Part model, mm, in its own coordinate system. A direction names the side the tool comes from. Coordinates: 2 decimals unless noted, no trailing zeros. Loops run counter-clockwise (first coordinate to the right, second up) from the corner with the lowest first, then second, coordinate; pieces in that order, holes last. Notation, with made-up numbers: (-38, 76.25) - (10, 76.25) arc R11 ccw to (10, 94.25) - close; hole circle Ø5 at (-16.5, 47.5). An arc over 180 degrees is marked (long way). Use a Markdown table: item, result. Add a question column.
1. 3-axis set-ups, long thin cutter, end or side, ignore diameter. For faces 5 (the flat face through (-19, -1, -12.8)), 6 (the flat face through (-20, -1, -36)), 7 (the flat face through (-1, -1, -6.4)): which of +Z, -Z, +X, -X, +Y, -Y reach the whole face in a straight line?
2. Band-saw the part on D-D, the plane z = -8. Give the cut face in (x, y), plus the area to 4 significant figures.
3. Band-saw the part on A-A, the plane z = -17.7. Give the cut face in (x, y).
4. Wall check: probe 1 along X at (y, z) = (-0.85, -30.5); probe 2 along Y at (x, z) = (-10, 0.8); probe 3 along Z at (x, y) = (-5, 7). Give the ranges that are in metal, low to high. Write a range as [from, to].
5. Band-saw the part on C-C, the plane x = -17.5. Count the separate pieces of the cut face and the enclosed holes in it, plus the area to 3 significant figures.
6. Band-saw the part on B-B, the plane y = 17. Give the cut face in (x, z), plus the area to 3 significant figures.
7. Pull direction Z, two halves, no side cores. Call faces 1 (the cylindrical face through (-3.65, -0.74, -33.56)), 2 (the flat face through (-10, 6, 1.5)), 3 (the cylindrical face through (-10, 20, 1)), 4 (the flat face through (-10, -1, -40)): pulls with the +Z half, pulls with the -Z half, needs draft (parallel to the pull), parting line crosses it, or undercut.
8. Drop flat-ended pins along their axis: pin 1 (1.6 mm diameter, centred on x = -1, y = -1, fed in from +Z); pin 2 (6 mm diameter, centred on x = -13, y = 11.5, fed in from -Z); pin 3 (0.8 mm diameter, centred on x = -0.5, y = -1, fed in from -Z). Give the stop position or say it passes through.
from build123d import *

# Parameters (mm, degrees)
BOSS_EXTRUDE1_DEPTH  = 20
CUT_EXTRUDE2_DEPTH   = 20
CUT_EXTRUDE3_DEPTH   = 20
SKETCH4_R            = 3.75
CUT_EXTRUDE4_DEPTH   = 20
SKETCH5_R            = 1.45
CUT_EXTRUDE5_DEPTH   = 20
CIRPATTERN1_COUNT    = 4
SKETCH6_R            = 1.6
CUT_EXTRUDE6_DEPTH   = 20
LPATTERN1_COUNT      = 6
LPATTERN1_PITCH      = 6.4
CUT_EXTRUDE7_DEPTH   = 20
LPATTERN2_COUNT      = 5
LPATTERN2_PITCH      = 6.4
MIRROR1_COPY_1_DEPTH = 20
MIRROR1_COPY_2_DEPTH = 20
MIRROR1_COPY_3_DEPTH = 20
MIRROR1_COPY_4_DEPTH = 20
FILLET3_R            = 3.65
FILLET4_R            = 3.65


with BuildPart() as part:
    # Sketch1 → Boss-Extrude1 (new body)
    with BuildSketch(Plane(origin=(0, 0, 0), x_dir=(0, 0, -1), z_dir=(1, 0, 0))):
        Polygon((0, 0), (0, 20), (-1.5, 20), (-1.5, -1.5), (40, -1.5), (40, 0), align=None)
    extrude(amount=-BOSS_EXTRUDE1_DEPTH)

    # Sketch2 → Cut-Extrude2 (cut)
    with BuildSketch(Plane(origin=(0, 0, 0), x_dir=(0, 0, -1), z_dir=(1, 0, 0))):
        with BuildLine():
            Line((-1.5, 0), (-1.5, -1.5))
            Line((-1.5, -1.5), (0, -1.5))
            ThreePointArc((0, -1.5), (-1.060660172, -1.060660172), (-1.5, 0))
        make_face()
    extrude(amount=-CUT_EXTRUDE2_DEPTH, mode=Mode.SUBTRACT)

    # Sketch3 → Cut-Extrude3 (cut)
    with BuildSketch(Plane.XY.offset(1.5)):
        with BuildLine():
            Line((-20, 10), (-20, 21.790535073))
            Line((-20, 21.790535073), (0, 21.790535073))
            Line((0, 21.790535073), (0, 10))
            ThreePointArc((0, 10), (-10, 20), (-20, 10))
        make_face()
    extrude(amount=-CUT_EXTRUDE3_DEPTH, mode=Mode.SUBTRACT)

    # Sketch4 → Cut-Extrude4 (cut)
    with BuildSketch(Plane.XY.offset(1.5)):
        with Locations((-10, 10)):
            Circle(SKETCH4_R)
    extrude(amount=-CUT_EXTRUDE4_DEPTH, mode=Mode.SUBTRACT)

    # Sketch5 → Cut-Extrude5 (cut)
    with BuildSketch(Plane.XY.offset(1.5)):
        with Locations((-10, 2.5)):
            Circle(SKETCH5_R)
    cut_extrude5 = extrude(amount=-CUT_EXTRUDE5_DEPTH, mode=Mode.SUBTRACT)

    # CirPattern1: Cut-Extrude5 ×4 about axis
    cirpattern1_axis = Axis((-10, 10, 0), (0, 0, 1))
    for i in range(1, CIRPATTERN1_COUNT):
        add(cut_extrude5.rotate(cirpattern1_axis, i * 360 / CIRPATTERN1_COUNT), mode=Mode.SUBTRACT)

    # Sketch6 → Cut-Extrude6 (cut)
    with BuildSketch(Plane(origin=(0, 0, 0), x_dir=(1, 0, 0), z_dir=(0, 1, 0))):
        with Locations(Location((-10, 4.9, 0), (0, 0, 270))):
            Circle(SKETCH6_R)
    cut_extrude6 = extrude(amount=-CUT_EXTRUDE6_DEPTH, mode=Mode.SUBTRACT)

    # LPattern1: Cut-Extrude6 ×6
    with Locations(*[(0, 0, -i * LPATTERN1_PITCH) for i in range(1, LPATTERN1_COUNT)]):
        add(cut_extrude6, mode=Mode.SUBTRACT)

    # Sketch7 → Cut-Extrude7 (cut)
    with BuildSketch(Plane(origin=(0, 0, 0), x_dir=(1, 0, 0), z_dir=(0, 1, 0))):
        with BuildLine():
            Line((0, 6.4), (-2.05, 6.4))
            ThreePointArc((-2.05, 6.4), (-3.65, 8), (-2.05, 9.6))
            Line((-2.05, 9.6), (0, 9.6))
            Line((0, 9.6), (0, 6.4))
        make_face()
    cut_extrude7 = extrude(amount=-CUT_EXTRUDE7_DEPTH, mode=Mode.SUBTRACT)

    # LPattern2: Cut-Extrude7 ×5
    with Locations(*[(0, 0, -i * LPATTERN2_PITCH) for i in range(1, LPATTERN2_COUNT)]):
        add(cut_extrude7, mode=Mode.SUBTRACT)

    # Mirror1: Cut-Extrude7 across plane
    add(cut_extrude7.mirror(Plane.ZY.offset(10)), mode=Mode.SUBTRACT)

    # Mirror1 copy 1 sketch → Mirror1 copy 1 (cut)
    with BuildSketch(Plane(origin=(-20, 0, -6.4), x_dir=(-1, 0, 0), z_dir=(0, 1, 0))):
        with BuildLine():
            Line((0, -6.4), (-2.05, -6.4))
            ThreePointArc((-2.05, -6.4), (-3.65, -8), (-2.05, -9.6))
            Line((-2.05, -9.6), (0, -9.6))
            Line((0, -9.6), (0, -6.4))
        make_face()
    extrude(amount=-MIRROR1_COPY_1_DEPTH, mode=Mode.SUBTRACT)

    # Mirror1 copy 2 sketch → Mirror1 copy 2 (cut)
    with BuildSketch(Plane(origin=(-20, 0, -12.8), x_dir=(-1, 0, 0), z_dir=(0, 1, 0))):
        with BuildLine():
            Line((0, -6.4), (-2.05, -6.4))
            ThreePointArc((-2.05, -6.4), (-3.65, -8), (-2.05, -9.6))
            Line((-2.05, -9.6), (0, -9.6))
            Line((0, -9.6), (0, -6.4))
        make_face()
    extrude(amount=-MIRROR1_COPY_2_DEPTH, mode=Mode.SUBTRACT)

    # Mirror1 copy 3 sketch → Mirror1 copy 3 (cut)
    with BuildSketch(Plane(origin=(-20, 0, -19.2), x_dir=(-1, 0, 0), z_dir=(0, 1, 0))):
        with BuildLine():
            Line((0, -6.4), (-2.05, -6.4))
            ThreePointArc((-2.05, -6.4), (-3.65, -8), (-2.05, -9.6))
            Line((-2.05, -9.6), (0, -9.6))
            Line((0, -9.6), (0, -6.4))
        make_face()
    extrude(amount=-MIRROR1_COPY_3_DEPTH, mode=Mode.SUBTRACT)

    # Mirror1 copy 4 sketch → Mirror1 copy 4 (cut)
    with BuildSketch(Plane(origin=(-20, 0, -25.6), x_dir=(-1, 0, 0), z_dir=(0, 1, 0))):
        with BuildLine():
            Line((0, -6.4), (-2.05, -6.4))
            ThreePointArc((-2.05, -6.4), (-3.65, -8), (-2.05, -9.6))
            Line((-2.05, -9.6), (0, -9.6))
            Line((0, -9.6), (0, -6.4))
        make_face()
    extrude(amount=-MIRROR1_COPY_4_DEPTH, mode=Mode.SUBTRACT)

    # Fillet3
    fillet3_edges = [part.edges().sort_by_distance(p)[0] for p in [
        (0, -0.75, -40),
    ]]
    fillet(fillet3_edges, radius=FILLET3_R)

    # Fillet4
    fillet4_edges = [part.edges().sort_by_distance(p)[0] for p in [
        (-20, -0.75, -40),
    ]]
    fillet(fillet4_edges, radius=FILLET4_R)


solid = part.part
Geometry check:
| question | item | result |
|---|---|---|
| 1 | face 5 | -X, +Y, -Y |
| 1 | face 6 | +Z, -Z, -X, +Y, -Y |
| 1 | face 7 | +X, +Y, -Y |
| 2 | outline | (-16.35, -1.5) - (-3.65, -1.5) - (-3.65, 0) - (-16.35, 0) - close |
| 2 | area | 19.05 mm^2 |
| 3 | outline | (-20, -1.5) - (-11.6, -1.5) - (-11.6, 0) - (-20, 0) - close; (-8.4, -1.5) - (0, -1.5) - (0, 0) - (-8.4, 0) - close |
| 4 | probe 1 | x = [-20, -11.6], [-8.4, 0] |
| 4 | probe 2 | y = [-1.27, 1.05], [3.95, 6.25], [13.75, 16.05], [18.95, 20] |
| 4 | probe 3 | z = [0, 1.5] |
| 5 | separate pieces | 7 |
| 5 | enclosed holes | 0 |
| 5 | area | 59.0 mm^2 |
| 6 | outline | (-17.14, 0) - (-11.36, 0) - (-11.36, 1.5) - (-17.14, 1.5) - close; (-8.64, 0) - (-2.86, 0) - (-2.86, 1.5) - (-8.64, 1.5) - close |
| 6 | area | 17.3 mm^2 |
| 7 | face 1 | undercut |
| 7 | face 2 | pulls with the +Z half |
| 7 | face 3 | needs draft |
| 7 | face 4 | pulls with the -Z half |
| 8 | pin 1 | stops at z = 1.49 |
| 8 | pin 2 | stops at z = 0 |
| 8 | pin 3 | stops at z = -38.75 |
